from build123d import *

# Parameters (mm, degrees)
SKETCH1_R           = 2.5
BOSS_EXTRUDE1_DEPTH = 4


with BuildPart() as part:
    # Sketch1 → Boss-Extrude1 (new body)
    with BuildSketch(Plane.XY):
        with BuildLine():
            Line((-20, -30), (-20, 40))
            Line((-20, 40), (0, 40))
            Line((0, 40), (0, 20))
            ThreePointArc((0, 20), (2.928932188, 12.928932188), (10, 10))
            Line((10, 10), (30, 10))
            Line((30, 10), (30, -30))
            Line((30, -30), (-20, -30))
        make_face()
        with Locations((-10, 32.5)):
            Circle(SKETCH1_R, mode=Mode.SUBTRACT)
        with Locations((-10, 0)):
            Circle(SKETCH1_R, mode=Mode.SUBTRACT)
        with Locations((-10, -20)):
            Circle(SKETCH1_R, mode=Mode.SUBTRACT)
        with Locations((20, 0)):
            Circle(SKETCH1_R, mode=Mode.SUBTRACT)
        with Locations((20, -20)):
            Circle(SKETCH1_R, mode=Mode.SUBTRACT)
        with Locations((-10, 20)):
            Circle(SKETCH1_R, mode=Mode.SUBTRACT)
    extrude(amount=BOSS_EXTRUDE1_DEPTH)


solid = part.part
Model file for the job. Use its own axes, mm. A direction names the side the tool comes from. Give positions to 0.01 mm unless a question says otherwise; leave off trailing zeros. Order: outer loops, then holes, each group sorted by start corner. A loop starts at its lowest first (then second) coordinate and runs counter-clockwise, first axis right, second up. Notation, with made-up numbers: (33.5, 76.25) -> (62.5, 76.25) arc R16 ccw to (62.5, 81.25) -> close; hole circle Ø8 at (-25, 50). An arc over 180 degrees is marked (long way). Use CSV: the item, a comma, the result in double quotes.
1. Mould opens along Y. For faces 3 (the flat face through (0, 30, 2)), 4 (the cylindrical face through (-10.33, 22.48, 1.97)), 5 (the cylindrical face through (-12.5, 0.1, 2)), 6 (the flat face through (5, -30, 2)) say: +Y half, -Y half, draft (parallel to the pull), parting line (faces both ways), or undercut.
Outcome:
face 3,"draft"
face 4,"undercut"
face 5,"undercut"
face 6,"-Y half"
2. Drill centre lines: line 1 along Y through (x, z) = (-10, 3); line 2 along Y through (x, z) = (20, 2.7); line 3 along Y through (x, z) = (21.5, 3.15). Where is each one in solid material? Low to high. Write a range as from..to.
Outcome:
line 1,"-30..-22.5, -17.5..-2.5, 2.5..17.5, 22.5..30, 35..40"
line 2,"-30..-22.5, -17.5..-2.5, 2.5..10"
line 3,"-30..-22, -18..-2, 2..10"
3. Band-saw the part on A-A, the plane x = 20. Give the cut face in (y, z), then the cut area to 3 significant figures.
Outcome:
outline,"(-30, 0) -> (-22.5, 0) -> (-22.5, 4) -> (-30, 4) -> close; (-17.5, 0) -> (-2.5, 0) -> (-2.5, 4) -> (-17.5, 4) -> close; (2.5, 0) -> (10, 0) -> (10, 4) -> (2.5, 4) -> close"
area,"120 mm²"
4. Band-saw the part on B-B, the plane y = 32.5. Give the cut face in (x, z), then the cut area to 3 significant figures.
Outcome:
outline,"(-20, 0) -> (-12.5, 0) -> (-12.5, 4) -> (-20, 4) -> close; (-7.5, 0) -> (0, 0) -> (0, 4) -> (-7.5, 4) -> close"
area,"60.0 mm²"
5. Drop flat-ended pins along their axis: pin 1 (2 mm diameter, centred on y = 27, z = 3, fed in from +X); pin 2 (6.5 mm diameter, centred on x = 20, y = 0, fed in from +Z); pin 3 (1 mm diameter, centred on x = 21, z = 2.5, fed in from +Y). Give the stop position or say it passes through.
Outcome:
pin 1,"x = 0"
pin 2,"z = 4"
pin 3,"y = 10"
6. Band-saw the part on C-C, the plane x = -10. Give the cut face in (y, z).
Outcome:
outline,"(-30, 0) -> (-22.5, 0) -> (-22.5, 4) -> (-30, 4) -> close; (-17.5, 0) -> (-2.5, 0) -> (-2.5, 4) -> (-17.5, 4) -> close; (2.5, 0) -> (17.5, 0) -> (17.5, 4) -> (2.5, 4) -> close; (22.5, 0) -> (30, 0) -> (30, 4) -> (22.5, 4) -> close; (35, 0) -> (40, 0) -> (40, 4) -> (35, 4) -> close"
7. Band-saw the part on D-D, the plane y = -20. Give the cut face in (x, z), then the cut area to 3 significant figures.
Outcome:
outline,"(-20, 0) -> (-12.5, 0) -> (-12.5, 4) -> (-20, 4) -> close; (-7.5, 0) -> (17.5, 0) -> (17.5, 4) -> (-7.5, 4) -> close; (22.5, 0) -> (30, 0) -> (30, 4) -> (22.5, 4) -> close"
area,"160 mm²"
8. 3-axis set-ups, long thin cutter, end or side, ignore diameter. For faces 1 (the cylindrical face through (17.5, -19.9, 2)), 2 (the flat face through (20, 10, 2)): which of +Z, -Z, +X, -X, +Y, -Y reach the whole face in a straight line?
Outcome:
face 1,"+Z, -Z"
face 2,"+Z, -Z, +X, +Y"
